from build123d import *

# Parameters (mm, degrees)
SKETCH1_R           = 5
SKETCH1_R_2         = 2
BOSS_EXTRUDE1_DEPTH = 50
CUT_EXTRUDE13_DEPTH = 16.5
BOSS_EXTRUDE2_DEPTH = 50
SKETCH13_R          = 1.9
CUT_EXTRUDE12_DEPTH = 23.5
CUT_EXTRUDE14_DEPTH = 16.5
SKETCH20_R          = 1.5
CUT_EXTRUDE15_DEPTH = 26


with BuildPart() as part:
    # Sketch1 → Boss-Extrude1 (new body)
    with BuildSketch(Plane.XY):
        with Locations((0, -20)):
            Circle(SKETCH1_R)
        with Locations((0, -20)):
            Circle(SKETCH1_R_2, mode=Mode.SUBTRACT)
        with BuildLine():
            Line((2.5, 24.874685928), (2.5, 14.790199458))
            ThreePointArc((2.5, 14.790199458), (14.947457842, -1.254393904), (0, -15))
            ThreePointArc((0, -15), (3.535533906, -16.464466094), (5, -20))
            ThreePointArc((5, -20), (3.535533906, -23.535533906), (0, -25))
            ThreePointArc((0, -25), (24.968651828, -1.251569376), (2.5, 24.874685928))
        make_face()
    extrude(amount=BOSS_EXTRUDE1_DEPTH)

    # Sketch16 → Cut-Extrude13 (cut)
    with BuildSketch(Plane.XY.offset(50)):
        with BuildLine():
            Line((0, -25.2), (5.2, -25.2))
            Line((5.2, -25.2), (5.2, -20))
            ThreePointArc((5.2, -20), (-3.676955262, -16.323044738), (0, -25.2))
        make_face()
    cut_extrude13 = extrude(amount=-CUT_EXTRUDE13_DEPTH, mode=Mode.SUBTRACT)

    # Mirror2: Cut-Extrude13 across plane
    add(cut_extrude13.mirror(Plane(origin=(0, 0, 25), x_dir=(1, 0, 0), z_dir=(0, 0, -1))), mode=Mode.SUBTRACT)

    # Sketch17 → Boss-Extrude2 (add)
    with BuildSketch(Plane(origin=(0, 0, 0), x_dir=(-1, 0, 0), z_dir=(0, 0, -1))):
        Polygon((-20.2, 24.8), (-11.15099728, 22.375327029), (-20.2, 0), (-11.15099728, -22.375327029), (-20.2, -24.8), (-25, -29.6), (-25, 29.6), align=None)
    extrude(amount=-BOSS_EXTRUDE2_DEPTH)

    # Sketch13 → Cut-Extrude12 (cut, through all)
    with BuildSketch(Plane.ZY.offset(-2.5)):
        with Locations((37.5, 19.832442693)):
            Circle(SKETCH13_R)
        with Locations((12.5, 19.832442693)):
            Circle(SKETCH13_R)
    extrude(amount=-CUT_EXTRUDE12_DEPTH, mode=Mode.SUBTRACT)

    # Sketch19 → Cut-Extrude14 (cut)
    with BuildSketch(Plane.XY.offset(50)):
        with BuildLine():
            Line((2.937921703, -15.709473684), (2.937921703, -14.709473684))
            ThreePointArc((2.937921703, -14.709473684), (2.090334438, -14.853635984), (1.235879849, -14.949))
            ThreePointArc((1.235879849, -14.949), (2.121257859, -15.252341093), (2.937921703, -15.709473684))
        make_face()
    cut_extrude14 = extrude(amount=-CUT_EXTRUDE14_DEPTH, mode=Mode.SUBTRACT)

    # Mirror4: Cut-Extrude14 across plane
    add(cut_extrude14.mirror(Plane(origin=(0, 0, 25), x_dir=(1, 0, 0), z_dir=(0, 0, -1))), mode=Mode.SUBTRACT)

    # Sketch20 → Cut-Extrude15 (cut, through all)
    with BuildSketch(Plane(origin=(0, 0, 0), x_dir=(0, 0, -1), z_dir=(1, 0, 0))):
        with Locations((-25, 0)):
            Circle(SKETCH20_R)
    extrude(amount=CUT_EXTRUDE15_DEPTH, mode=Mode.SUBTRACT)


solid = part.part
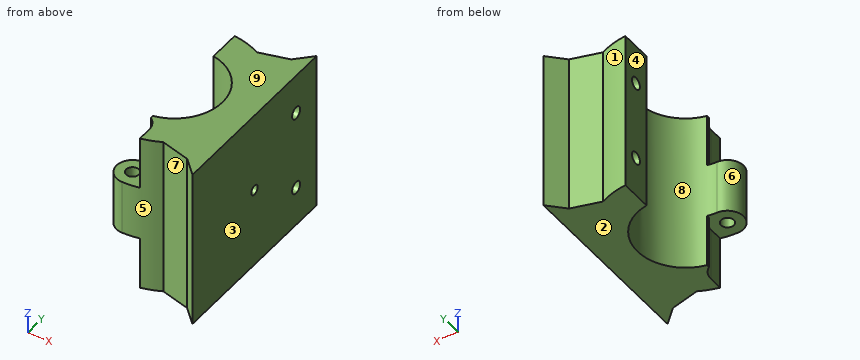
Design review of the part built by this model. Coordinates are the model's own, in mm. Face numbers are marked on the shaded views. A direction names the side the tool comes from. Coordinates: 2 decimals unless noted, no trailing zeros. Order: outer loops, then holes, each group sorted by start corner. A loop starts at its lowest first (then second) coordinate and runs counter-clockwise, first axis right, second up.
Item 1: Take a section at C-C, the plane z = 12.5. Write out the cut boundary in (x, y), then the cut area to 3 significant figures.
Item 2: Take a section at B-B, the plane y = 0. Write out the cut boundary in (x, z).
Item 3: The part is to be moulded in two halves that separate along Y. For the marked faces 6, 7, 8 and 9, say which applies: pulls with the +Y half, pulls with the -Y half, needs draft (parallel to the pull), parting line crosses it, or undercut.
Item 4: For pin 1 Ø6 at (x, z) = (10, 20) entering from -Y; pin 2 Ø5 at (x, y) = (1, -19.5) entering from -Z; pin 3 Ø1.3 at (y, z) = (-21.5, 39.5) entering from -X, all flat-tipped, find the tip position at first contact; note any pin that passes through.
Item 5: For line 1 (X direction, y = -20, z = 20); line 2 (X direction, y = 17.5, z = 4); line 3 (Z direction, x = 1.5, y = -22.5), list the stretches that pass through material, from the lowest coordinate up.
Item 6: Take a section at D-D, the plane x = 10. Write out the cut boundary in (y, z).
Item 7: Take a section at A-A, the plane z = 25. Write out the cut boundary in (x, y).
Item 8: For the marked faces 1, 2, 3, 4 and 5, list the 3-axis set-ups (+Z, -Z, +X, -X, +Y, -Y) from which the entire face can be reached by the end or side of a thin tool; tool diameter is ignored.
The answers:
1. outline: (2.5, 14.79) arc R15 cw to (2.94, -14.71) - (2.94, -15.71) arc R5.2 cw to (5.2, -20) - (5.2, -24.45) arc R25 ccw to (11.15, -22.38) - (20.2, -24.8) - (25, -29.6) - (25, 17.93) - (2.5, 17.93) - close; (2.5, 21.73) - (25, 21.73) - (25, 29.6) - (20.2, 24.8) - (11.15, 22.38) arc R25 ccw to (2.5, 24.87) - close
1. area: 716 mm2
2. outline: (15, 0) - (25, 0) - (25, 23.5) - (15, 23.5) - close; (15, 26.5) - (25, 26.5) - (25, 50) - (15, 50) - close
3. face 6: parting line crosses it
3. face 7: pulls with the -Y half
3. face 8: undercut
3. face 9: needs draft
4. pin 1: stops at y = -24
4. pin 2: stops at z = 16.5
4. pin 3: stops at x = 5.2
5. line 1: x = -5 to -2, 2 to 25
5. line 2: x = 2.5 to 25
5. line 3: z = 16.5 to 33.5
6. outline: (-22.91, 0) - (-11.18, 0) - (-11.18, 50) - (-22.91, 50) - close; (11.18, 0) - (22.91, 0) - (22.91, 50) - (11.18, 50) - close; hole circle Ø3.8 at (19.83, 12.5); hole circle Ø3.8 at (19.83, 37.5)
7. outline: (0, -25) arc R25 ccw to (11.15, -22.38) - (20.2, -24.8) - (25, -29.6) - (25, -1.5) - (14.92, -1.5) arc R15 cw to (0, -15) arc R5 ccw to start; (2.5, 14.79) arc R15 cw to (14.92, 1.5) - (25, 1.5) - (25, 29.6) - (20.2, 24.8) - (11.15, 22.38) arc R25 ccw to (2.5, 24.87) - close; hole circle Ø4 at (0, -20)
8. face 1: +Z, -Z, +Y
8. face 2: -Z, +X, -X, +Y, -Y
8. face 3: +Z, -Z, +X, +Y, -Y
8. face 4: +Z, -Z, -X, +Y
8. face 5: +Z, -Z, -Y
